Job drawing, mm, ordinate dimensions from the low corner. One solid piece. A direction names the side the tool comes from. Coordinates: 2 decimals unless noted, no trailing zeros. Loops run counter-clockwise (first coordinate to the right, second up) from the corner with the lowest first, then second, coordinate; pieces in that order, holes last. Notation, with made-up numbers: (32, -19) -> (65, -19) arc R15 ccw to (65, -13) -> close; hole circle Ø7 at (-2, -10.75). An arc over 180 degrees is marked (long way). Use one line per item in the form item = value. Start each with the question number.
(1) Drill centre lines: L1, parallel to Y at x = 41, z = 32.5; L2, parallel to X at y = 111, z = 29.5; L3, parallel to Z at x = 19, y = 126 (3 decimals). Where is each one in solid material? Low to high. Write a range as [from, to].
(2) Mould opens along Y. For the marked faces 1, 2 and 3 say: +Y half, -Y half, draft (parallel to the pull), parting line (faces both ways), or undercut.
(3) 3-axis set-ups, long thin cutter, end or side, ignore diameter. For the marked faces 4, 5 and 6: which of +Z, -Z, +X, -X, +Y, -Y reach the whole face in a straight line?
(4) Band-saw the part on C-C on z = 8.5. Give the cut face in (x, y).
(5) Pin check, flat tips, straight feed: P1, Ø1, axis at x = 111, y = 81, coming from the +Z side (3 decimals); P2, Ø8, axis at y = 26.5, z = 10.5, coming from the +X side; P3, Ø1, axis at x = 25.5, y = 174, coming from the -Z side (3 decimals). Stop position of each tip, or through.
(6) Band-saw the part on B-B on y = 52.5. Give the cut face in (x, z) (1 decimal).
(7) Band-saw the part on A-A on x = 29.5. Give the cut face in (y, z) (3 decimals).
(8) Band-saw the part on D-D on y = 126. Give the cut face in (x, z) (3 decimals), then the cut area to 3 significant figures.
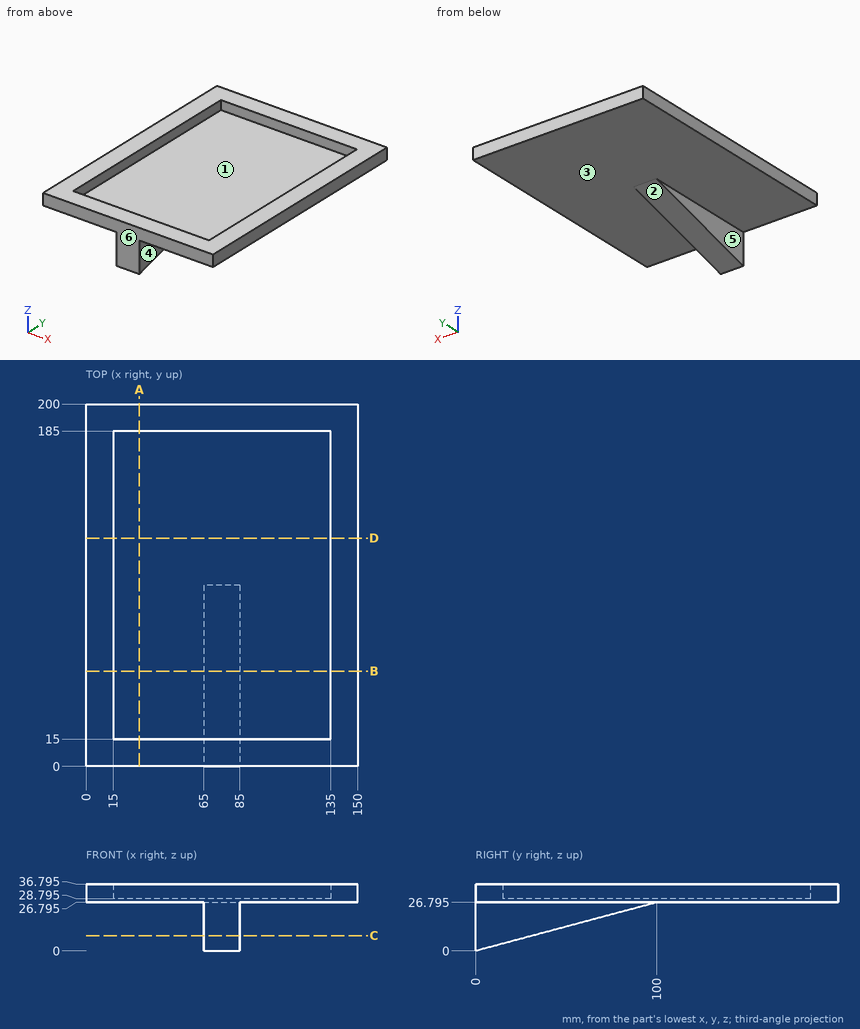
A:
q1.L1 = [0, 15], [185, 200]
q1.L2 = [0, 15], [135, 150]
q1.L3 = [26.795, 28.795]
q2.face_1 = undercut
q2.face_2 = +Y half
q2.face_3 = draft
q3.face_4 = -Z, +X, +Y, -Y
q3.face_5 = -Z, -X, +Y, -Y
q3.face_6 = +Z, -Z, +X, -X, -Y
q4.outline = (65, 0) -> (85, 0) -> (85, 31.72) -> (65, 31.72) -> close
q5.P1 = 28.795
q5.P2 = 85
q5.P3 = 26.795
q6.outline = (0, 26.8) -> (65, 26.8) -> (65, 14.1) -> (85, 14.1) -> (85, 26.8) -> (150, 26.8) -> (150, 36.8) -> (135, 36.8) -> (135, 28.8) -> (15, 28.8) -> (15, 36.8) -> (0, 36.8) -> close
q7.outline = (0, 26.795) -> (200, 26.795) -> (200, 36.795) -> (185, 36.795) -> (185, 28.795) -> (15, 28.795) -> (15, 36.795) -> (0, 36.795) -> close
q8.outline = (0, 26.795) -> (150, 26.795) -> (150, 36.795) -> (135, 36.795) -> (135, 28.795) -> (15, 28.795) -> (15, 36.795) -> (0, 36.795) -> close
q8.area = 540 mm²
